```python
from build123d import *

# Parameters (mm, degrees)
EXTRUDE_1_DEPTH     = 20
SKETCH_2_R          = 1.5
CUT_EXTRUDE_1_DEPTH = 20
SKETCH_3_R          = 2.5
CUT_EXTRUDE_2_DEPTH = 20


with BuildPart() as part:
    # 草图1 → 凸台-拉伸1 (new body)
    with BuildSketch(Plane.XY):
        with BuildLine():
            Line((-28, 0), (-21, 0))
            ThreePointArc((-21, 0), (0, 21), (21, 0))
            Line((21, 0), (28, 0))
            ThreePointArc((28, 0), (0, 28), (-28, 0))
        make_face()
    extrude(amount=EXTRUDE_1_DEPTH)

    # 草图2 → 切除-拉伸1 (cut)
    with BuildSketch(Plane.XZ):
        with Locations((-24, 5)):
            Circle(SKETCH_2_R)
        with Locations((-24, 15)):
            Circle(SKETCH_2_R)
    cut_extrude_1 = extrude(amount=-CUT_EXTRUDE_1_DEPTH, mode=Mode.SUBTRACT)

    # 镜向1: 切除-拉伸1 across plane
    add(cut_extrude_1.mirror(Plane(origin=(0, 0, 0), x_dir=(0, 0, 1), z_dir=(1, 0, 0))), mode=Mode.SUBTRACT)

    # 草图3 → 切除-拉伸2 (cut)
    with BuildSketch(Plane(origin=(0, 5, 0), x_dir=(-1, 0, 0), z_dir=(0, -1, 0))):
        with Locations((24, -5)):
            Circle(SKETCH_3_R)
        with Locations((24, -15)):
            Circle(SKETCH_3_R)
    cut_extrude_2 = extrude(amount=-CUT_EXTRUDE_2_DEPTH, mode=Mode.SUBTRACT)

    # 镜向2: 切除-拉伸2 across plane
    add(cut_extrude_2.mirror(Plane(origin=(0, 0, 0), x_dir=(0, 0, 1), z_dir=(1, 0, 0))), mode=Mode.SUBTRACT)


solid = part.part
```
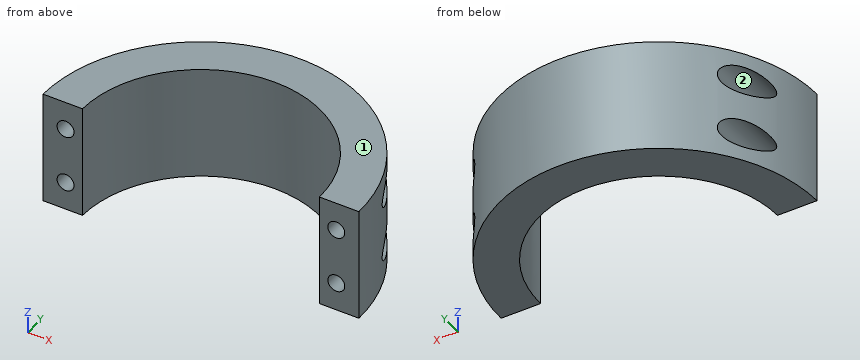
Geometry check sheet. Reference: the model listing, model coordinates, mm. Face numbers are marked on the shaded views. A direction names the side the tool comes from. Give positions to 0.01 mm unless a question says otherwise; leave off trailing zeros. Order: outer loops, then holes, each group sorted by start corner. A loop starts at its lowest first (then second) coordinate and runs counter-clockwise, first axis right, second up.
1. Section check C-C, the plane x = -24. Enter the section's corners in (y, z), and give its area (3 significant figures).
2. Access from +Z, -Z, +X, -X, +Y, -Y to the whole of each face (thin tool, end or side, straight path). Record for the marked faces 1 and 2.
3. Gauge pin test, flat ends, axial feed: pin 1 Ø3 at (x, z) = (19.5, 9.5) entering from +Y; pin 2 Ø3 at (x, z) = (4, 17) entering from -Y; pin 3 Ø4 at (x, z) = (-23.5, 5.5) entering from +Y; pin 4 Ø2.5 at (x, z) = (-24, 15) entering from -Y. Record the tip position at first contact, or that the pin passes through.
4. Section check D-D, the plane y = 12.5. Enter the section's corners in (x, z).
5. Section check A-A, the plane y = 7.25. Enter the section's corners in (x, z), and give its area (3 significant figures).
6. Section check B-B, the plane z = 5. Enter the section's corners in (x, y).
7. Thickness scan on L1, parallel to Z at x = 24, y = 9; L2, parallel to Z at x = -24, y = 2.95; L3, parallel to X at y = 12, z = 15. Record the ranges inside material, lowest first.
Values follow:
1. outline: (0, 0) - (14.42, 0) - (14.42, 2.5) - (5, 2.5) - (5, 3.5) - (0, 3.5) - close; (0, 6.5) - (5, 6.5) - (5, 7.5) - (14.42, 7.5) - (14.42, 12.5) - (5, 12.5) - (5, 13.5) - (0, 13.5) - close; (0, 16.5) - (5, 16.5) - (5, 17.5) - (14.42, 17.5) - (14.42, 20) - (0, 20) - close
1. area: 164 mm2
2. face 1: +Z, +X, -X, +Y, -Y
2. face 2: +Y
3. pin 1: stops at y = 21.45
3. pin 2: stops at y = 20.27
3. pin 3: stops at y = 17.94
3. pin 4: passes through
4. outline: (-25.05, 0) - (-16.87, 0) - (-16.87, 20) - (-25.05, 20) - (-25.05, 17.27) arc R2.5 cw (long way) to (-25.05, 12.73) - (-25.05, 7.27) arc R2.5 cw (long way) to (-25.05, 2.73) - close; (16.87, 0) - (25.05, 0) - (25.05, 2.73) arc R2.5 cw (long way) to (25.05, 7.27) - (25.05, 12.73) arc R2.5 cw (long way) to (25.05, 17.27) - (25.05, 20) - (16.87, 20) - close
5. outline: (-27.05, 0) - (-19.71, 0) - (-19.71, 20) - (-27.05, 20) - close; (19.71, 0) - (27.05, 0) - (27.05, 20) - (19.71, 20) - close; hole circle Ø5 at (-24, 5); hole circle Ø5 at (-24, 15); hole circle Ø5 at (24, 5); hole circle Ø5 at (24, 15)
5. area: 215 mm2
6. outline: (-28, 0) - (-25.5, 0) - (-25.5, 5) - (-26.5, 5) - (-26.5, 9.04) arc R28 ccw to start; (-22.5, 0) - (-21, 0) arc R21 cw to (21, 0) - (22.5, 0) - (22.5, 5) - (21.5, 5) - (21.5, 17.94) arc R28 ccw to (-21.5, 17.94) - (-21.5, 5) - (-22.5, 5) - close; (25.5, 0) - (28, 0) arc R28 ccw to (26.5, 9.04) - (26.5, 5) - (25.5, 5) - close
7. L1: z = 0 to 2.5, 7.5 to 12.5, 17.5 to 20
7. L2: z = 0 to 3.5, 6.5 to 13.5, 16.5 to 20
7. L3: x = -21.5 to -17.23, 17.23 to 21.5
